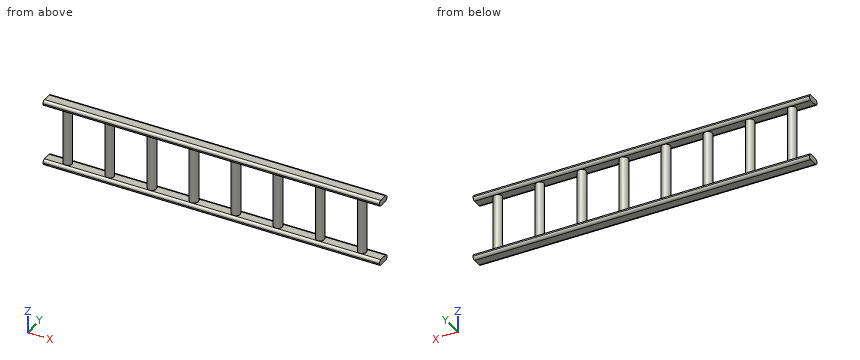
```python
from build123d import *

# Parameters (mm, degrees)
SKETCH3_W           = 150
SKETCH3_H           = 50
BOSS_EXTRUDE1_DEPTH = 20
SKETCH4_R           = 15
BOSS_EXTRUDE2_DEPTH = 200
SKETCH5_W           = 150
SKETCH5_H           = 50
BOSS_EXTRUDE3_DEPTH = 20
FILLET2_R           = 10


with BuildPart() as part:
    # Sketch3 → Boss-Extrude1 (new body)
    with BuildSketch(Plane.XY):
        Rectangle(SKETCH3_W, SKETCH3_H)
    extrude(amount=BOSS_EXTRUDE1_DEPTH)

    # Sketch4 → Boss-Extrude2 (add)
    with BuildSketch(Plane.XY.offset(20)):
        Circle(SKETCH4_R)
    extrude(amount=BOSS_EXTRUDE2_DEPTH)

    # Sketch5 → Boss-Extrude3 (add)
    with BuildSketch(Plane.XY.offset(220)):
        Rectangle(SKETCH5_W, SKETCH5_H)
    extrude(amount=BOSS_EXTRUDE3_DEPTH)

    # Mirror1: part across plane


with BuildPart() as part_1:
    add(part.part)
    add(part.part.mirror(Plane(origin=(75, -25, 20), x_dir=(0, 0, 1), z_dir=(-1, 0, 0))))

    # Mirror2: part across plane


with BuildPart() as part_2:
    add(part_1.part)
    add(part_1.part.mirror(Plane(origin=(225, 25, 240), x_dir=(0, 0, 1), z_dir=(-1, 0, 0))))

    # Mirror3: part across plane


with BuildPart() as part_3:
    add(part_2.part)
    add(part_2.part.mirror(Plane(origin=(525, 25, 240), x_dir=(0, 0, 1), z_dir=(-1, 0, 0))))

    # Fillet2
    fillet2_edges = [part_3.edges().sort_by_distance(p)[0] for p in [
        (525, -25, 20),
        (525, -25, 0),
        (525, 25, 0),
        (525, 25, 20),
        (525, 25, 220),
        (525, 25, 240),
        (525, -25, 220),
        (525, -25, 240),
    ]]
    fillet(fillet2_edges, radius=FILLET2_R - 0.0001)  # a hair under: the kernel refuses the full size


solid = part_3.part
```
Verification items for the finished model (mm, model axes). Round coordinates to 2 decimals unless told otherwise and drop trailing zeros. Write each loop counter-clockwise with the first axis right and the second up, starting at its lowest first coordinate (ties: lowest second). Pieces come first, ordered by that corner, then holes. Notation, with made-up numbers: (-9.75, 35) -> (5.25, 35) arc R11 cw to (5.25, 43) -> close; hole circle Ø10 at (7, 60). An arc over 180 degrees is marked (long way). Write each question's results on one line, items separated by ' | '. Start each with the question number.
1. Cross-section at A-A (z = 200). Enter the section's corners in (x, y).
2. Depth check by flat-ended pin: P1, Ø2, axis at x = 141, z = 180, coming from the -Y side; P2, Ø12, axis at x = 872.5, y = 19.5, coming from the +Z side; P3, Ø1, axis at y = 4, z = 172, coming from the +X side. Enter the tip coordinate at first touch or a pass-through.
3. Material ranges on probe 1 along Z at (x, y) = (33.5, -17); probe 2 along Z at (x, y) = (497, 14); probe 3 along Y at (x, z) = (1004.5, 225.5), recorded low to high. Write a range as from..to.
Solutions:
1) outline: circle Ø30 at (0, 0); circle Ø30 at (150, 0); circle Ø30 at (300, 0); circle Ø30 at (450, 0); circle Ø30 at (600, 0); circle Ø30 at (750, 0); circle Ø30 at (900, 0); circle Ø30 at (1050, 0)
2) P1: stops at y = -12.69 | P2: stops at z = 240 | P3: stops at x = 1064.59
3) probe 1: z = 0.2..19.8, 220.2..239.8 | probe 2: z = 0..20, 220..240 | probe 3: y = -23.93..23.93
